from build123d import *

# Parameters (mm, degrees)
SKETCH_1_W          = 20
SKETCH_1_H          = 20
EXTRUDE_1_DEPTH     = 2
SKETCH_2_W          = 20
SKETCH_2_H          = 2
EXTRUDE_2_DEPTH     = 18
SKETCH_4_R          = 1.5
CUT_EXTRUDE_1_DEPTH = 18
SKETCH_6_R          = 1.5
CUT_EXTRUDE_2_DEPTH = 18


with BuildPart() as part:
    # 草图1 → 凸台-拉伸1 (new body)
    with BuildSketch(Plane.XY):
        Rectangle(SKETCH_1_W, SKETCH_1_H)
    extrude(amount=EXTRUDE_1_DEPTH)

    # 草图2 → 凸台-拉伸2 (add)
    with BuildSketch(Plane.XY.offset(2)):
        with Locations((0, -9)):
            Rectangle(SKETCH_2_W, SKETCH_2_H)
    extrude(amount=EXTRUDE_2_DEPTH)

    # 草图4 → 切除-拉伸1 (cut)
    with BuildSketch(Plane.XZ.offset(10)):
        with Locations((-5, 10)):
            Circle(SKETCH_4_R)
        with Locations((5, 10)):
            Circle(SKETCH_4_R)
    extrude(amount=-CUT_EXTRUDE_1_DEPTH, mode=Mode.SUBTRACT)

    # 草图6 → 切除-拉伸2 (cut)
    with BuildSketch(Plane(origin=(0, 0, 0), x_dir=(-1, 0, 0), z_dir=(0, 0, -1))):
        with Locations((5, 0)):
            Circle(SKETCH_6_R)
        with Locations((-5, 0)):
            Circle(SKETCH_6_R)
    extrude(amount=-CUT_EXTRUDE_2_DEPTH, mode=Mode.SUBTRACT)


solid = part.part
Check sheet for the modelled part. Datum: model origin and axes. Units: mm. A direction names the side the tool comes from. Give positions to 0.01 mm unless a question says otherwise; leave off trailing zeros. Loops run counter-clockwise (first coordinate to the right, second up) from the corner with the lowest first, then second, coordinate; pieces in that order, holes last. Notation, with made-up numbers: M -21.5,75.5 L 4.5,75.5 A22 ccw 4.5,98.5 Z; hole C 65.5,84.5 d6. An arc over 180 degrees is marked long. Answer as a JSON object with one key per item and string values. Group by question number.
Q1. Cross-section at D-D on z = 13.25. Record the cut outline in (x, y), then the cut area to 3 significant figures.
Q2. Cross-section at C-C on y = 5.75. Record the cut outline in (x, z), then the cut area to 3 significant figures.
Q3. Cross-section at A-A on z = 10. Record the cut outline in (x, y).
Q4. Cross-section at B-B on x = 5. Record the cut outline in (y, z).
Q5. Material ranges on line 1 along Y through (x, z) = (5, 0.75); line 2 along Z through (x, y) = (-5, -8.55); line 3 along Z through (x, y) = (-8.5, 4.25), recorded low to high. Write a range as [from, to].
Q6. Go/stop test with flat-tipped pins: P1, Ø1.5, axis at x = -5, z = 15, coming from the +Y side; P2, Ø10, axis at x = -5.5, z = 4, coming from the +Y side; P3, Ø5, axis at x = 5, y = 0, coming from the +Z side. Record where each tip stops, or that it passes through.
Q7. Release check for a two-part mould opening along X. For faces 1 (the flat face through (0, 0, 0)), 2 (the flat face through (10, -8.2, 5.5)), 3 (the cylindrical face through (-6.386, -0.575, 0.986)) record: released by +X, released by -X, zero draft, split by the parting line, or undercut.
Q8. Access from +Z, -Z, +X, -X, +Y, -Y to the whole of each face (thin tool, end or side, straight path). Record for faces 4 (the flat face through (0, -8, 11)), 5 (the flat face through (0, 10, 1)).
Evaluation:
{
 "1": {"outline": "M -10,-10 L 10,-10 L 10,-8 L -10,-8 Z", "area": "40.0 mm2"},
 "2": {"outline": "M -10,0 L 10,0 L 10,2 L -10,2 Z", "area": "40.0 mm2"},
 "3": {"outline": "M -10,-10 L -6.5,-10 L -6.5,-8 L -10,-8 Z; M -3.5,-10 L 3.5,-10 L 3.5,-8 L -3.5,-8 Z; M 6.5,-10 L 10,-10 L 10,-8 L 6.5,-8 Z"},
 "4": {"outline": "M -10,0 L -1.5,0 L -1.5,2 L -8,2 L -8,8.5 L -10,8.5 Z; M -10,11.5 L -8,11.5 L -8,20 L -10,20 Z; M 1.5,0 L 10,0 L 10,2 L 1.5,2 Z"},
 "5": {"line 1": "y = [-10, -1.5], [1.5, 10]", "line 2": "z = [0, 8.5], [11.5, 20]", "line 3": "z = [0, 2]"},
 "6": {"P1": "stops at y = -8", "P2": "stops at y = 10", "P3": "stops at z = 2"},
 "7": {"face 1": "zero draft", "face 2": "released by +X", "face 3": "undercut"},
 "8": {"face 4": "+Z, +X, -X, +Y", "face 5": "+Z, -Z, +X, -X, +Y"}
}
